Build history of the part. All positions in model axes, mm. Face numbers are marked on the shaded views. A direction names the side the tool comes from. Give positions to 0.01 mm unless a question says otherwise; leave off trailing zeros. Write each loop counter-clockwise with the first axis right and the second up, starting at its lowest first coordinate (ties: lowest second). Pieces come first, ordered by that corner, then holes. Notation, with made-up numbers: M 34,12 L 50,12 A24 ccw 50,45 Z; hole C -12.5,-18 d5. An arc over 180 degrees is marked long. One line per item, written item: value. Start each with the question number.
from build123d import *

# Parameters (mm, degrees)
F1_DEPTH = 63.5
F2_DEPTH = 25.4
F3_DEPTH = 7.9375
F5_R     = 6.35
F6_R     = 12.7
F7_DEPTH = 76.201
F8_SIZE  = 2.54


with BuildPart() as f1:
    # F0 (on Front) → F1 (new body, symmetric)
    with BuildSketch(Plane.XZ):
        Polygon((-41.275, 9.525), (-41.275, -9.525), (41.275, -9.525), (41.275, 9.525), (22.225, 9.525), align=None)
    extrude(amount=F1_DEPTH, both=True)

    # F0 (on Front) → F2 (join, symmetric)
    with BuildSketch(Plane.XZ):
        with BuildLine():
            Line((22.225, 9.525), (41.275, 9.525))
            Line((41.275, 9.525), (41.275, 27.0002))
            ThreePointArc((41.275, 27.0002), (45.9246798487, 38.2255201513), (57.15, 42.8752))
            Line((57.15, 42.8752), (60.325, 42.8752))
            Line((60.325, 42.8752), (85.4920223873, 42.8752))
            Line((85.4920223873, 42.8752), (85.4920223873, 61.9252))
            Line((85.4920223873, 61.9252), (60.325, 61.9252))
            Line((60.325, 61.9252), (57.15, 61.9252))
            ThreePointArc((57.15, 61.9252), (32.4542956671, 51.6959043329), (22.225, 27.0002))
            Line((22.225, 27.0002), (22.225, 9.525))
        make_face()
    extrude(amount=F2_DEPTH, both=True)

    # F0 (on Front) → F3 (join, symmetric)
    with BuildSketch(Plane.XZ):
        with BuildLine():
            add(Edge.make_bspline(
                [(-41.275, 9.525), (-40.758330375, 43.9411401749), (18.6435300857, 61.9299374521), (57.15, 61.9252)],
                knots=[0, 0, 0, 0, 111.5045361635, 111.5045361635, 111.5045361635, 111.5045361635], degree=3))
            Line((-41.275, 9.525), (22.225, 9.525))
            Line((22.225, 9.525), (22.225, 27.0002))
            ThreePointArc((22.225, 27.0002), (32.4542956671, 51.6959043329), (57.15, 61.9252))
        make_face()
    extrude(amount=F3_DEPTH, both=True)

    # F0 (on Front) → F4 (revolve)
    with BuildSketch(Plane.XZ):
        Polygon((85.4920223873, 66.675), (85.4920223873, 61.9252), (85.4920223873, 42.8752), (85.4920223873, 38.1), (111.125, 38.1), (111.125, 66.675), align=None)
    revolve(axis=Axis((85.4920223873, 0, 52.4002), (0, 0, 1)))

    # F5
    f5_edges = [f1.edges().sort_by_distance(p)[0] for p in [
        (-41.275, -63.5, 0),
        (41.275, -63.5, 0),
        (41.275, 63.5, 0),
        (-41.275, 63.5, 0),
    ]]
    fillet(f5_edges, radius=F5_R)

    # F6 (on face) → F7 (cut, through all)
    with BuildSketch(Plane.XY.offset(66.675)):
        with Locations((85.4920223873, 0)):
            Circle(F6_R)
    extrude(amount=-F7_DEPTH, mode=Mode.SUBTRACT)

    # F8
    f8_edges = [f1.edges().sort_by_distance(p)[0] for p in [
        (72.792022, 0, 66.675),
        (72.792022, 0, 38.1),
    ]]
    chamfer(f8_edges, length=F8_SIZE)


solid = f1.part
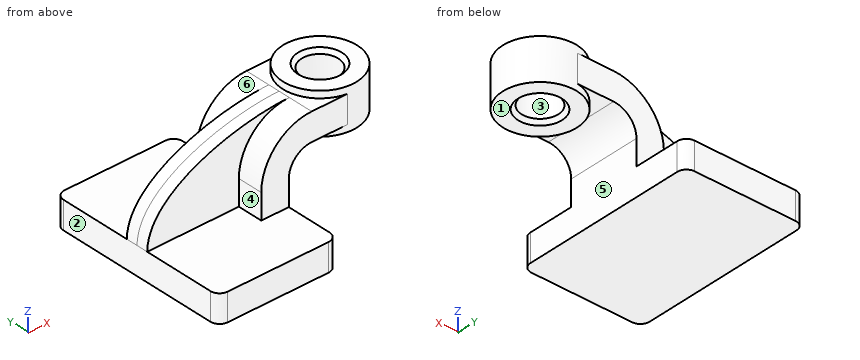
1) Band-saw the part on A-A (y = -21). List the corners of the cut face in (x, z) (3 decimals).
2) Probe line 1 along Z through (x, y) = (17, 56) (3 decimals); line 2 along Z through (x, y) = (68, -6) (3 decimals); line 3 along X through (y, z) = (24.5, -3) (3 decimals). List the from-to ranges inside material, lowest first. Write a range as from..to.
3) Drop flat-ended pins along their axis: P1, Ø12, axis at x = 24, z = 24, coming from the -Y side; P2, Ø12, axis at x = 8.5, y = -39.5, coming from the +Z side (3 decimals); P3, Ø6, axis at x = 33.5, y = 8, coming from the +Z side. Give the stop position or say it passes through.
4) Mould opens along X. For the marked faces 1, 2 and 3 say: released by +X, released by -X, zero draft, split by the parting line, or undercut.
5) Tool access for the marked faces 4, 5 and 6: list every direction of +Z, -Z, +X, -X, +Y, -Y with a clear straight run to the whole face (end or side of a thin tool).
6) Band-saw the part on B-B (y = 54). List the corners of the cut face in (x, z) (3 decimals).
Model answer:
1. outline: M -41.275,-9.525 L 41.275,-9.525 L 41.275,27 A15.875 cw 57.15,42.875 L 70.793,42.875 L 70.793,38.1 L 100.191,38.1 L 100.191,66.675 L 70.793,66.675 L 70.793,61.925 L 57.15,61.925 A34.925 ccw 22.225,27 L 22.225,9.525 L -41.275,9.525 Z
2. line 1: z = -9.525..9.525
2. line 2: z = 38.1..66.675
2. line 3: x = -41.275..41.275
3. P1: stops at y = -25.4
3. P2: stops at z = 9.525
3. P3: stops at z = 60.43
4. face 1: zero draft
4. face 2: released by -X
4. face 3: undercut
5. face 4: +Z, -X, -Y
5. face 5: -Z, +X, +Y, -Y
5. face 6: +Z, -X, +Y
6. outline: M -41.275,-9.525 L 41.275,-9.525 L 41.275,9.525 L -41.275,9.525 Z
